Autodesk Fusion 360 part; units mm, degrees
sketch "Sketch1" plane through (0, 0, 0) normal (0, 1, 0) x (1, 0, 0)
  circle A0 centre (0, 0) radius 30
  circle A1 centre (0, 0) radius 4
  dimension "d1" = 60
  dimension "d3" = 8
extrude "Extrude1" add sketch "Sketch1" along normal blind 60
chamfer "Chamfer1" distance 20 angle 45 1 edges at (-27.9698, 60, 10.8485) measured on face at (21.2216, 60, 1.4904)
sketch "Sketch2" plane through (0, 0, 0) normal (0, 1, 0) x (1, 0, 0)
  circle A0 centre (0, 0) radius 11
  dimension "d8" = 22
extrude "Extrude2" cut sketch "Sketch2" along normal blind 8
extrude "Extrude3" cut 1 faces at (23.514, 0, 2.0369) along direction (0, 1, 0) blind 38
extrude "Extrude4" cut 1 faces at (8.6257, 8, 0.5465) along direction (0, 1, 0) blind 38
extrude "Extrude5" add 1 faces at (8.6257, 46, 0.5465) along direction (0, -1, 0) blind 0.5
chamfer "Chamfer2" distance 7 angle 45 1 edges at (-3.7293, 45.5, 1.4465) measured on face at (8.6257, 45.5, 0.5465)
chamfer "Chamfer3" distance 2 angle 45 1 edges at (-10.2556, 38, -3.9778) measured on face at (10.9453, 43, 1.0952)
chamfer "Chamfer4" distance 1 angle 45 1 edges at (-3.7293, 60, -1.4465) measured on face at (7.9479, 60, 0.6955)
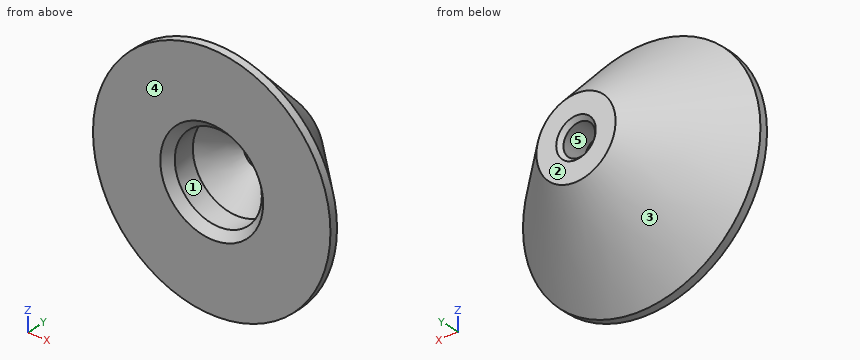
Check sheet for the modelled part. Datum: model origin and axes. Units: mm. Face numbers are marked on the shaded views. A direction names the side the tool comes from. Coordinates: 2 decimals unless noted, no trailing zeros. Loops run counter-clockwise (first coordinate to the right, second up) from the corner with the lowest first, then second, coordinate; pieces in that order, holes last.
1) Material ranges on probe 1 along X at (y, z) = (57, 0); probe 2 along Z at (x, y) = (0, 54.75), recorded low to high.
2) Sectioned sample at D-D (y = 50). Record the boundary of the cut face in (x, z), and give its area (3 significant figures).
3) Sectioned sample at C-C (y = 43). Record the boundary of the cut face in (x, z), and give its area (3 significant figures).
4) Access from +Z, -Z, +X, -X, +Y, -Y to the whole of each face (thin tool, end or side, straight path). Record for the marked faces 1 and 2.
5) Gauge pin test, flat ends, axial feed: pin 1 (5 mm diameter, centred on y = 55, z = -6.5, fed in from -X); pin 2 (10 mm diameter, centred on x = -8, y = 43.5, fed in from -Z); pin 3 (24 mm diameter, centred on x = 2.5, z = -2, fed in from -Y); pin 4 (9 mm diameter, centred on x = 0, z = 0, fed in from -Y). Record the tip position at first contact, or that the pin passes through.
6) Release check for a two-part mould opening along X. For the marked faces 3, 4 and 5 record: released by +X, released by -X, zero draft, split by the parting line, or undercut.
Check sheet entries:
1. probe 1: x = -13 to -4, 4 to 13
1. probe 2: z = -15.25 to -4, 4 to 15.25
2. outline: circle Ø40 at (0, 0); hole circle Ø13 at (0, 0)
2. area: 1,120 mm2
3. outline: circle Ø54 at (0, 0); hole circle Ø22 at (0, 0)
3. area: 1,910 mm2
4. face 1: -Y
4. face 2: +Z, -Z, +X, -X, +Y
5. pin 1: stops at x = -16.41
5. pin 2: stops at z = -29.67
5. pin 3: stops at y = 38
5. pin 4: stops at y = 52
6. face 3: split by the parting line
6. face 4: zero draft
6. face 5: undercut
